Autodesk Inventor part; units mm, degrees
ref_plane "YZ Plane" through (0, 0, 0) normal (1, 0, 0) x (0, 1, 0)
ref_plane "XZ Plane" through (0, 0, 0) normal (0, 1, 0) x (-1, 0, 0)
ref_plane "XY Plane" through (0, 0, 0) normal (0, 0, 1) x (1, 0, 0)
sketch "Schizzo1" plane through (0, 0, 0) normal (0, 1, 0) x (-1, 0, 0)
  line L0 (30, 32) -> (-30, 32)
  line L1 (-30, 32) -> (-30, -32)
  line L2 (-30, -32) -> (30, -32)
  line L3 (30, -32) -> (30, 32)
  line L4 (0, 0) -> (41.9471, 0) construction
  line L5 (0, 0) -> (0, -48.4274) construction
  line L6 (28.8, 32) -> (28.8, 29.75) construction
  line L7 (28.8, 29.75) -> (30, 29.75) construction
  line L8 (28.8, 29.75) -> (28.1, 29.75) construction
  circle A0 centre (28.1, 29.75) radius 0.35
  line L9 (28.8, -32) -> (28.8, -29.75) construction
  line L10 (28.8, -29.75) -> (30, -29.75) construction
  line L11 (28.8, -29.75) -> (28.1, -29.75) construction
  circle A1 centre (28.1, -29.75) radius 0.7
  circle A2 centre (28.1, -29.75) radius 0.35
  circle A3 centre (28.1, 29.75) radius 0.65
  line L12 (30, 31) -> (-30, 31)
  line L13 (-30, 31) -> (-30, -31)
  line L14 (-30, -31) -> (30, -31)
  line L15 (30, -31) -> (30, 31)
  dimension "d0" = 60
  dimension "d1" = 64
  dimension "d2" = 2.25
  dimension "d3" = 1.2
  dimension "d4" = 0.7
  dimension "d5" = 0.7
  dimension "d8" = 1.3
  dimension "d9" = 62
extrude "Estrusione1" add sketch "Schizzo1" along normal blind 1 contours L3 L12 L1 L0 | L3 L14 L1 L12 | L3 L2 L1 L14 | A0 | A1 | A2 | A3
extrude "Estrusione2" add sketch "Schizzo1" against normal blind 2.7 contours L3 L12 L1 L0 | L3 L2 L1 L14
sketch "Schizzo2" plane through (30, 0, 31) normal (0, 0, -1) x (-1, 0, 0)
  line L0 (0, -2.7) -> (60, -2.7)
  line L1 (0, -2.7) -> (0, 1) construction
  line L2 (0, -0.5) -> (6.4394, -0.5) construction
  line L3 (0, -0.5) -> (0, -0.65) construction
  line L4 (0, -0.65) -> (0, -2.15) construction
  line L5 (0, -2.15) -> (1, -2.15) construction
  line L6 (1, -2.15) -> (1.7, -2.15) construction
  circle A0 centre (1.7, -2.15) radius 0.7
  circle A1 centre (1.7, -2.15) radius 0.4
  line L7 (0, -0.5) -> (0, 0) construction
  point P0 (30, 0)
  dimension "d14" = 2.2
  dimension "d15" = 0.15
  dimension "d16" = 1.5
  dimension "d17" = 1
  dimension "d18" = 0.7
  dimension "d19" = 1.4
  dimension "d20" = 0.8
extrude "Estrusione3" add sketch "Schizzo2" along normal blind 2.2 contours A0 L0 | L0 A0 | A1
extrude "Estrusione4" cut sketch "Schizzo2" along normal blind 1.9
sketch "Schizzo3" plane through (-30, 0, -31) normal (0, 0, 1) x (1, 0, 0)
  line L0 (60, -2.7) -> (60, 1)
  line L1 (0, -2.7) -> (60, -2.7)
  line L2 (60, 0) -> (60, -0.65) construction
  line L3 (60, -0.65) -> (60, -2.15) construction
  line L4 (60, -2.15) -> (59, -2.15) construction
  line L5 (59, -2.15) -> (58.3, -2.15) construction
  circle A0 centre (58.3, -2.15) radius 0.7
  circle A1 centre (58.3, -2.15) radius 0.4
  line L6 (0, 0) -> (60, 0)
  point P0 (30, 0)
  dimension "d26" = 0.65
  dimension "d27" = 1.5
  dimension "d28" = 1
  dimension "d29" = 0.7
  dimension "d30" = 1.4
  dimension "d31" = 0.8
extrude "Estrusione5" add sketch "Schizzo3" along normal blind 2.2 contours A0 L1 | L1 A0 | A1
extrude "Estrusione6" cut sketch "Schizzo3" along normal blind 1.9
properties part number "coperchio contieni SD"
Input: part model. Units: mm. Frame: model coordinates. A direction names the side the tool comes from. Round coordinates to 2 decimals unless told otherwise and drop trailing zeros. Loops run counter-clockwise (first coordinate to the right, second up) from the corner with the lowest first, then second, coordinate; pieces in that order, holes last. Notation, with made-up numbers: M 63.25,-30.5 L 76.25,-30.5 A22 cw 76.25,2.5 Z; hole C 29.5,64.25 d4. An arc over 180 degrees is marked long. Answer in a Markdown table with one row per item. Add a question column.
1. Set-up query: faces 4 (the face through (28, -2, -28.8)), 5 (the face through (-30, 0.4, -0.1)), 6 (the face through (28.68, -2.74, -28.95)). Return all of +Z, -Z, +X, -X, +Y, -Y with unobstructed straight access to the full face (end or side cutting, diameter ignored); none if empty.
2. Section A-A (x = 25). Output: boundary loops of the cut face in (y, z).
3. Section B-B (z = 5). Output: boundary loops of the cut face in (x, y).
4. Ray query, probe 1 along Z at (x, y) = (-24, -1.9); probe 2 along Y at (x, z) = (13.5, 17.5). Return the intervals inside material, ascending.
5. Contact query for flat-ended pins moving along their axis: pin 1 (8 mm diameter, centred on x = -12.5, z = -19, fed in from -Y); pin 2 (0.8 mm diameter, centred on x = -4, z = -31.5, fed in from -Y); pin 3 (2 mm diameter, centred on y = -2.5, z = -6.5, fed in from +X). Output: stop coordinate, or through.
6. Mould query, pull axis Z, two halves, no side actions, for faces 1 (the face through (0, -1, 32)), 2 (the face through (0, -1, -32)), 3 (the face through (0, -1, -31)). Classes: released by +Z, released by -Z, zero draft, split by the parting line, or undercut.
Values follow:
| question | item | result |
|---|---|---|
| 1 | face 4 | +X, -X, -Y |
| 1 | face 5 | +Z, -Z, -X, +Y, -Y |
| 1 | face 6 | none |
| 2 | outline | M -2.7,-32 L 1,-32 L 1,32 L -2.7,32 L -2.7,31 L 0,31 L 0,-31 L -2.7,-31 Z |
| 3 | outline | M -30,0 L 30,0 L 30,1 L -30,1 Z |
| 4 | probe 1 | -32 to -31, 31 to 32 |
| 4 | probe 2 | 0 to 1 |
| 5 | pin 1 | y = 0 |
| 5 | pin 2 | y = -2.7 |
| 5 | pin 3 | through |
| 6 | face 1 | released by +Z |
| 6 | face 2 | released by -Z |
| 6 | face 3 | undercut |
